Autodesk Inventor part; units mm, degrees
ref_plane "YZ Plane" through (0, 0, 0) normal (1, 0, 0) x (0, 1, 0)
ref_plane "XZ Plane" through (0, 0, 0) normal (0, 1, 0) x (-1, 0, 0)
ref_plane "XY Plane" through (0, 0, 0) normal (0, 0, 1) x (1, 0, 0)
sketch "Sketch1" plane through (0, 0, 0) normal (0, 0, 1) x (1, 0, 0)
  line L0 (0, 0) -> (0, 20)
  line L1 (0, 20) -> (6, 20)
  line L2 (6, 20) -> (6, 6)
  line L3 (6, 6) -> (66, 6)
  line L4 (66, 6) -> (66, 0)
  line L5 (66, 0) -> (0, 0)
  dimension "d0" = 20
  dimension "d1" = 6
  dimension "d2" = 14
  dimension "d3" = 60
  dimension "d4" = 6
extrude "Extrusion1" add sketch "Sketch1" along normal blind 40
sketch "Sketch2" plane through (6, 6, 0) normal (0, 1, 0) x (1, 0, 0)
  line L0 (0, 0) -> (0, -40)
  circle A0 centre (47, -20) radius 6.35
  line L1 (60, 0) -> (0, 0)
  line L2 (60, -40) -> (0, -40)
  point P0 (-6, 0)
  dimension "d8" = 12.7
extrude "Extrusion2" cut sketch "Sketch2" against normal blind 40
properties part number "motor_angle"
The listing builds one solid part. Answer for the finished solid, in the listing's coordinates (mm). A direction names the side the tool comes from. Give positions to 0.01 mm unless a question says otherwise; leave off trailing zeros. Loops run counter-clockwise (first coordinate to the right, second up) from the corner with the lowest first, then second, coordinate; pieces in that order, holes last. Notation, with made-up numbers: (65.5, 32) - (90.5, 32) arc R31 cw to (90.5, 58) - close; hole circle Ø10 at (6, 59.5). An arc over 180 degrees is marked (long way). Return JSON: item names as keys, results as strings. Group by question number.
1. Given pin 1 Ø6 at (y, z) = (6.5, 6) entering from +X; pin 2 Ø12 at (x, z) = (32, 22) entering from +Y; pin 3 Ø4 at (y, z) = (16.5, 8.5) entering from +X, each flat-ended and moving along its own axis, determine where each tip first touches the part or whether it passes through.
2. Find section D-D (z = 31.5). Write down the section's boundary in (x, y).
3. Which of the six approach directions +Z, -Z, +X, -X, +Y, -Y give full straight-line access (tool end or side, diameter ignored) to faces 4 (the flat face through (36, 6, 20)), 5 (the flat face through (66, 3, 20))?
4. Find section C-C (y = 2). Write down the section's boundary in (x, z), then the cut area to 3 significant figures.
5. Determine the mould class of faces 1 (the flat face through (3, 20, 20)), 2 (the cylindrical face through (47.96, 3.04, 23.86)), 3 (the flat face through (25.2, 5.7, 0)) for opening direction Z: pulls with the +Z half, pulls with the -Z half, needs draft (parallel to the pull), parting line crosses it, or undercut.
6. Straight lines are drawn through the part: line 1 (X direction, y = 1.55, z = 20); line 2 (Z direction, x = 53, y = 2.25); line 3 (Y direction, x = 27, z = 11). For each, find the intervals that lie inside material, in ascending order. Write a range as [from, to].
7. Find section B-B (z = 20). Write down the section's boundary in (x, y).
8. Find section A-A (x = 53). Write down the section's boundary in (y, z), then the cut area to 3 significant figures.
Verdict:
{
 "1": {"pin 1": "stops at x = 66", "pin 2": "stops at y = 6", "pin 3": "stops at x = 6"},
 "2": {"outline": "(0, 0) - (66, 0) - (66, 6) - (6, 6) - (6, 20) - (0, 20) - close"},
 "3": {"face 4": "+Z, -Z, +X, +Y", "face 5": "+Z, -Z, +X, +Y, -Y"},
 "4": {"outline": "(0, 0) - (66, 0) - (66, 40) - (0, 40) - close; hole circle Ø12.7 at (53, 20)", "area": "2,510 mm^2"},
 "5": {"face 1": "needs draft", "face 2": "undercut", "face 3": "pulls with the -Z half"},
 "6": {"line 1": "x = [0, 46.65], [59.35, 66]", "line 2": "z = [0, 13.65], [26.35, 40]", "line 3": "y = [0, 6]"},
 "7": {"outline": "(0, 0) - (46.65, 0) - (46.65, 6) - (6, 6) - (6, 20) - (0, 20) - close; (59.35, 0) - (66, 0) - (66, 6) - (59.35, 6) - close"},
 "8": {"outline": "(0, 0) - (6, 0) - (6, 13.65) - (0, 13.65) - close; (0, 26.35) - (6, 26.35) - (6, 40) - (0, 40) - close", "area": "164 mm^2"}
}
